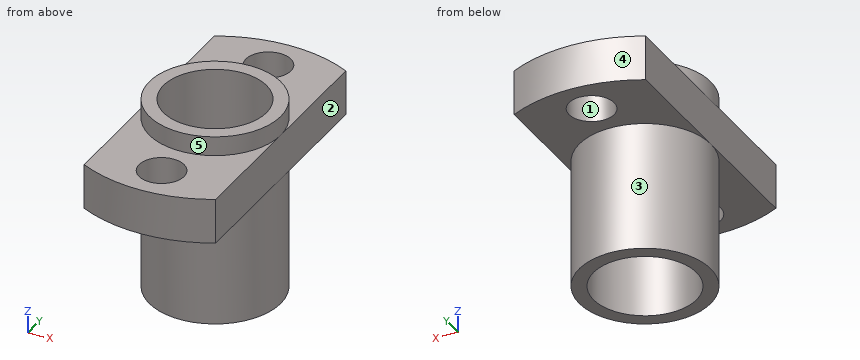
```python
from build123d import *

# Parameters (mm, degrees)
SKETCH_1_R          = 11
EXTRUDE_1_DEPTH     = 3.5
CUT_EXTRUDE_1_REACH = 17.945
SKETCH_3_R          = 5.1
EXTRUDE_2_DEPTH     = 1.5
EXTRUDE_START       = 10
SKETCH_4_R          = 5.1
EXTRUDE_3_DEPTH     = 10
CUT_EXTRUDE_2_REACH = 20.146
SKETCH_5_R          = 1.75
CUT_EXTRUDE_3_REACH = 21.288
SKETCH_6_R          = 4


with BuildPart() as part:
    # 草图1 → 凸台-拉伸1 (new body)
    with BuildSketch(Plane.XY):
        Circle(SKETCH_1_R)
    extrude(amount=EXTRUDE_1_DEPTH)

    # 草图2 → 切除-拉伸1 (cut, up to next)
    with BuildSketch(Plane.XY.offset(3.5), mode=Mode.PRIVATE) as cut_extrude_1_sk1:
        with BuildLine():
            ThreePointArc((-5.1, 9.746281342), (-11, 0), (-5.1, -9.746281342))
            Line((-5.1, -9.746281342), (-5.1, 9.746281342))
        make_face()
    cut_extrude_1_tool1 = extrude(cut_extrude_1_sk1.sketch, amount=-CUT_EXTRUDE_1_REACH, mode=Mode.PRIVATE) & part.part
    # 草图2 → 切除-拉伸1 (cut, up to next)
    with BuildSketch(Plane.XY.offset(3.5), mode=Mode.PRIVATE) as cut_extrude_1_sk2:
        with BuildLine():
            Line((5.1, 9.746281342), (5.1, -9.746281342))
            ThreePointArc((5.1, -9.746281342), (9.410100956, -5.696490147), (11, 0))
            ThreePointArc((11, 0), (9.410100956, 5.696490147), (5.1, 9.746281342))
        make_face()
    cut_extrude_1_tool2 = extrude(cut_extrude_1_sk2.sketch, amount=-CUT_EXTRUDE_1_REACH, mode=Mode.PRIVATE) & part.part
    add(cut_extrude_1_tool1.solids().sort_by_distance((-7.524361, 0, 3.5))[0], mode=Mode.SUBTRACT)
    add(cut_extrude_1_tool2.solids().sort_by_distance((7.524361, 0, 3.5))[0], mode=Mode.SUBTRACT)

    # 草图3 → 凸台-拉伸2 (add)
    with BuildSketch(Plane.XY.offset(3.5)):
        Circle(SKETCH_3_R)
    extrude(amount=EXTRUDE_2_DEPTH)

    # 草图4 → 凸台-拉伸3 (add)
    with BuildSketch(Plane(origin=(0, 0, 0), x_dir=(-1, 0, 0), z_dir=(0, 0, -1)).offset(EXTRUDE_START)):
        with Locations(Location((0, 0, 0), (0, 0, 180))):
            Circle(SKETCH_4_R)
    extrude(amount=-EXTRUDE_3_DEPTH)

    # 草图5 → 切除-拉伸2 (cut, up to next)
    with BuildSketch(Plane.XY.offset(3.5), mode=Mode.PRIVATE) as cut_extrude_2_sk1:
        with Locations((0, 8)):
            Circle(SKETCH_5_R)
    cut_extrude_2_tool1 = extrude(cut_extrude_2_sk1.sketch, amount=-CUT_EXTRUDE_2_REACH, mode=Mode.PRIVATE) & part.part
    # 草图5 → 切除-拉伸2 (cut, up to next)
    with BuildSketch(Plane.XY.offset(3.5), mode=Mode.PRIVATE) as cut_extrude_2_sk2:
        with Locations((0, -8)):
            Circle(SKETCH_5_R)
    cut_extrude_2_tool2 = extrude(cut_extrude_2_sk2.sketch, amount=-CUT_EXTRUDE_2_REACH, mode=Mode.PRIVATE) & part.part
    add(cut_extrude_2_tool1.solids().sort_by_distance((0, 8, 3.5))[0], mode=Mode.SUBTRACT)
    add(cut_extrude_2_tool2.solids().sort_by_distance((0, -8, 3.5))[0], mode=Mode.SUBTRACT)

    # 草图6 → 切除-拉伸3 (cut, up to next)
    with BuildSketch(Plane.XY.offset(5), mode=Mode.PRIVATE) as cut_extrude_3_sk1:
        Circle(SKETCH_6_R)
    cut_extrude_3_tool1 = extrude(cut_extrude_3_sk1.sketch, amount=-CUT_EXTRUDE_3_REACH, mode=Mode.PRIVATE) & part.part
    add(cut_extrude_3_tool1.solids().sort_by_distance((0, 0, 5))[0], mode=Mode.SUBTRACT)


solid = part.part
```
For this review, take the finished solid that the model builds, in its own axes (mm). Face numbers are marked on the shaded views. A direction names the side the tool comes from. Round coordinates to 2 decimals unless told otherwise and drop trailing zeros. Order: outer loops, then holes, each group sorted by start corner. A loop starts at its lowest first (then second) coordinate and runs counter-clockwise, first axis right, second up.
Q1. We need section B-B, the plane x = -2.75. Give the boundary of the cut face in (y, z), plus the area to 3 significant figures.
Findings below:
outline: (-10.65, 0) - (-4.3, 0) - (-4.3, -10) - (-2.9, -10) - (-2.9, 5) - (-4.3, 5) - (-4.3, 3.5) - (-10.65, 3.5) - close; (2.9, -10) - (4.3, -10) - (4.3, 0) - (10.65, 0) - (10.65, 3.5) - (4.3, 3.5) - (4.3, 5) - (2.9, 5) - close
area: 86.2 mm2
Q2. We need section D-D, the plane x = 0. Give the boundary of the cut face in (y, z), plus the area to 3 significant figures.
Findings below:
outline: (-11, 0) - (-9.75, 0) - (-9.75, 3.5) - (-11, 3.5) - close; (-6.25, 0) - (-5.1, 0) - (-5.1, -10) - (-4, -10) - (-4, 5) - (-5.1, 5) - (-5.1, 3.5) - (-6.25, 3.5) - close; (4, -10) - (5.1, -10) - (5.1, 0) - (6.25, 0) - (6.25, 3.5) - (5.1, 3.5) - (5.1, 5) - (4, 5) - close; (9.75, 0) - (11, 0) - (11, 3.5) - (9.75, 3.5) - close
area: 49.8 mm2
Q3. Wall thickness on line 1 (Y direction, x = 0, z = 1.6); line 2 (Y direction, x = 0, z = -5.75); line 3 (Z direction, x = 3.75, y = -5): over which ranges is each line inside the solid? List them lowest first.
Findings below:
line 1: y = -11 to -9.75, -6.25 to -4, 4 to 6.25, 9.75 to 11
line 2: y = -5.1 to -4, 4 to 5.1
line 3: z = 0 to 3.5
Q4. We need section A-A, the plane y = -8. Give the boundary of the cut face in (x, z).
Findings below:
outline: (-5.1, 0) - (-1.75, 0) - (-1.75, 3.5) - (-5.1, 3.5) - close; (1.75, 0) - (5.1, 0) - (5.1, 3.5) - (1.75, 3.5) - close
Q5. Machinability: for the marked faces 4 and 5, which of the approach directions +Z, -Z, +X, -X, +Y, -Y give a long, thin tool a straight path to every point of the face, cutting with its end or side? Answer none if there is none.
Findings below:
face 4: +Z, -Z, +Y
face 5: +Z
Q6. Insertion check: P1, Ø3, axis at x = 1.5, y = 7, coming from the +Z side; P2, Ø6, axis at x = 3.5, z = 1, coming from the +Y side; P3, Ø1, axis at x = -2, z = -4.5, coming from the +Y side. Each pin has a flat end and moves straight along its axis. Give the tip position at first contact, or say it passes through.
Findings below:
P1: stops at z = 3.5
P2: stops at y = 10.99
P3: stops at y = 4.87
Q7. Mouldability with a two-part tool opening along Y and no side actions: class the marked faces 1, 2 and 3 as pulls with the +Y half, pulls with the -Y half, needs draft (parallel to the pull), parting line crosses it, or undercut.
Findings below:
face 1: undercut
face 2: needs draft
face 3: parting line crosses it
Q8. We need section C-C, the plane z = 0.25. Give the boundary of the cut face in (x, y), plus the area to 3 significant figures.
Findings below:
outline: (-5.1, -9.75) arc R11 ccw to (5.1, -9.75) - (5.1, 9.75) arc R11 ccw to (-5.1, 9.75) - close; hole circle Ø8 at (0, 0); hole circle Ø3.5 at (0, -8); hole circle Ø3.5 at (0, 8)
area: 147 mm2
